from build123d import *

# Parameters (mm, degrees)
BOSS_EXTRUDE1_DEPTH  = 40
BOSS_EXTRUDE2_START  = -20
BOSS_EXTRUDE2_DEPTH  = 5
FILLET1_R            = 10
FILLET2_R            = 3
M4_CLEARANCE_HOLE1_D = 4.5
BOSS_EXTRUDE3_REACH  = 42
CHAMFER1_SIZE        = 0.5


with BuildPart() as part:
    # Sketch1 → Boss-Extrude1 (new body)
    with BuildSketch(Plane(origin=(0, 0, 0), x_dir=(1, 0, 0), z_dir=(0, 1, 0))):
        Polygon((0, 0), (0, -45), (5, -45), (5, -5), (45, -5), (45, 0), align=None)
    extrude(amount=-BOSS_EXTRUDE1_DEPTH)

    # Sketch2 → Boss-Extrude2 (add)
    with BuildSketch(Plane.XZ.offset(40).offset(BOSS_EXTRUDE2_START)):
        Polygon((5, 45), (25, 45), (25, 25), (45, 25), (45, 5), (5, 5), align=None)
    extrude(amount=-BOSS_EXTRUDE2_DEPTH)

    # Fillet1
    fillet1_edges = [part.edges().sort_by_distance(p)[0] for p in [
        (25, -17.5, 45),
        (45, -17.5, 25),
        (45, 0, 2.5),
        (2.5, 0, 45),
    ]]
    fillet(fillet1_edges, radius=FILLET1_R)

    # Fillet2
    fillet2_edges = [part.edges().sort_by_distance(p)[0] for p in [
        (0, -20, 0),
        (22.5, -40, 0),
        (0, -40, 22.5),
    ]]
    fillet(fillet2_edges, radius=FILLET2_R)

    # M4 Clearance Hole1 (through all)
    with Locations(Plane(origin=(0, -15, 0), x_dir=(1, 0, 0), z_dir=(0, 1, 0))):
        with Locations((35, -15), (15, -35)):
            Hole(M4_CLEARANCE_HOLE1_D / 2)

    # Sketch5 → Boss-Extrude3 (add, up to next)
    with BuildSketch(Plane(origin=(0, 0, 0), x_dir=(1, 0, 0), z_dir=(0, 1, 0)), mode=Mode.PRIVATE) as boss_extrude3_sk1:
        with BuildLine():
            Line((5, -25), (5, -5))
            Line((5, -5), (25, -5))
            ThreePointArc((25, -5), (19.142135624, -19.142135624), (5, -25))
        make_face()
    boss_extrude3_tool1 = extrude(boss_extrude3_sk1.sketch, amount=-BOSS_EXTRUDE3_REACH, mode=Mode.PRIVATE) - part.part
    add(boss_extrude3_tool1.solids().sort_by_distance((13.488264, 0, 13.488264))[0])

    # Chamfer1
    chamfer1_edges = [part.edges().sort_by_distance(p)[0] for p in [
        (4, -40, 45),
        (45, -40, 4),
        (0.878679656, -39.121320344, 45),
        (45, -39.121320344, 0.878679656),
        (0, -23.5, 45),
        (45, -23.5, 0),
        (0, -2.928932188, 42.071067812),
        (42.071067812, -2.928932188, 0),
        (0, 0, 19),
        (0.878679656, 0, 0.878679656),
        (19, 0, 0),
        (5, -12.5, 45),
        (45, -12.5, 5),
        (5, -2.928932188, 42.071067812),
        (42.071067812, -2.928932188, 5),
        (5, 0, 30),
        (30, 0, 5),
        (19.142135624, 0, 19.142135624),
    ]]
    chamfer(chamfer1_edges, length=CHAMFER1_SIZE)


solid = part.part
Read the model definition and answer for the solid it produces. Units are mm, in the model's axes. A direction names the side the tool comes from. Give positions to 0.01 mm unless a question says otherwise; leave off trailing zeros. Write each loop counter-clockwise with the first axis right and the second up, starting at its lowest first coordinate (ties: lowest second). Pieces come first, ordered by that corner, then holes. Notation, with made-up numbers: (49, 74.25) -> (65, 74.25) arc R5 cw to (65, 79.25) -> close; hole circle Ø1 at (61, 82.5). An arc over 180 degrees is marked (long way). Answer as a JSON object with one key per item and string values. Group by question number.
1) Consider L1, parallel to Z at x = 35, y = -18.6; L2, parallel to Y at x = 7, z = 6.5. Determine where each line is inside the solid, lowest interval first. Write a range as from..to.
2) Find section B-B (y = -24.5). Write down the section's boundary in (x, z), and give its area (3 significant figures).
3) Each of these flat-tipped pins is pushed along its axis until it touches: P1, Ø7.5, axis at x = 38, y = -10.5, coming from the +Z side; P2, Ø12, axis at x = 32.5, z = 26, coming from the -Y side; P3, Ø8, axis at y = -28.5, z = 21, coming from the +X side. Where does it stop, or does it pass through?
4) A tool of negligible diameter and unlimited length cuts with its end or side. For faces 4 (the flat face through (25, -18, 30)), 5 (the flat face through (21, -20, 21)), 6 (the flat face through (5, -8, 35)), from which of +Z, -Z, +X, -X, +Y, -Y can it reach the whole face along a straight path? Write none if from no direction.
5) Find section A-A (x = 32). Write down the section's boundary in (y, z), and give its area (3 significant figures).
6) The mould has two halves that part along Z. Classify faces 1 (the flat face through (25, -15, 21)), 2 (the flat face through (25, -30, 5)), 3 (the cylindrical face through (32.92, -17.53, 15.86)): +Z half, -Z half, draft (parallel to the pull), parting line (faces both ways), or undercut.
Values follow:
{
 "1": {"L1": "z = 0..12.75, 17.25..25", "L2": "y = -20..0"},
 "2": {"outline": "(0, 3) arc R3 ccw to (3, 0) -> (44.5, 0) -> (45, 0.5) -> (45, 5) -> (5, 5) -> (5, 45) -> (0.5, 45) -> (0, 44.5) -> close", "area": "423 mm2"},
 "3": {"P1": "stops at z = 5", "P2": "stops at y = -20", "P3": "stops at x = 5"},
 "4": {"face 4": "+Z, +X, +Y, -Y", "face 5": "+Z, +X, -Y", "face 6": "+Z, +X, +Y"},
 "5": {"outline": "(-40, 3) arc R3 ccw to (-37, 0) -> (-0.5, 0) -> (0, 0.5) -> (0, 4.5) -> (-0.5, 5) -> (-15, 5) -> (-15, 25) -> (-20, 25) -> (-20, 5) -> (-40, 5) -> close", "area": "298 mm2"},
 "6": {"face 1": "draft", "face 2": "+Z half", "face 3": "undercut"}
}
